The listing builds one solid part. Answer for the finished solid, in the listing's coordinates (mm). Face numbers are marked on the shaded views. Give positions to 0.01 mm unless a question says otherwise; leave off trailing zeros. Order: outer loops, then holes, each group sorted by start corner. A loop starts at its lowest first (then second) coordinate and runs counter-clockwise, first axis right, second up. Notation, with made-up numbers: (12, -26.75) - (39, -26.75) arc R29 ccw to (39, 12.25) - close; hole circle Ø4 at (-2.5, 80.5). An arc over 180 degrees is marked (long way). Answer as CSV lines item,"result". Start each with the question number.
1. Section A-A on y = 39 is taken. Give the vertices of the cut face in (x, z), and give its area (3 significant figures).
2. Flat-ended cylindrical pins translate along their axes: pin 1 (5.5 mm diameter, centred on x = -25.79, y = 74.34, fed in from +Z); pin 2 (7 mm diameter, centred on x = 26.21, y = -42.5, fed in from -Z). Find the tip coordinate at first contact, or state that the pin passes through.
3. Section B-B on z = 3 is taken. Give the vertices of the cut face in (x, y).
4. Section C-C on y = -69 is taken. Give the vertices of the cut face in (x, z), and give its area (3 significant figures).
5. Determine the mould class of the marked faces 1, 2 and 3 for opening direction X: +X half, -X half, draft (parallel to the pull), parting line (faces both ways), or undercut.
6. Consider line 1 along Y through (x, z) = (7, 7); line 2 along X through (y, z) = (32, 7.75); line 3 along Y through (x, z) = (-25.5, 7.5). Determine where each line is inside the solid, lowest interval first. Write a range as [from, to].
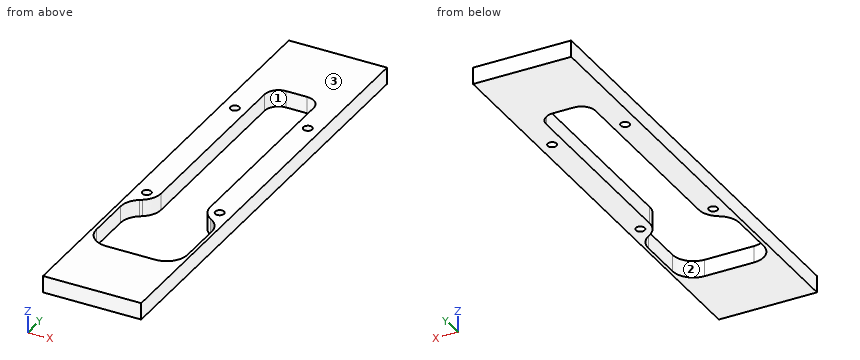
from build123d import *

# Parameters (mm, degrees)
F0_W     = 70
F0_H     = 326
F0_W_2   = 17
F0_H_2   = 17
F0_R     = 3.15
F1_DEPTH = 12
F2_R     = 15
F3_R     = 10


with BuildPart() as f1:
    # F0 (on Top) → F1 (new body)
    with BuildSketch(Plane.XY):
        Rectangle(F0_W, F0_H)
        Polygon((32.7086956522, -112.1642902674), (17.7086956522, -112.1642902674), (-17.2913043478, -112.1642902674), (-32.2913043478, -112.1642902674), (-32.2913043478, -57.1642902674), (-34.2913043478, -47.1642902674), (-34.2913043478, -32.1642902674), (-17.2913043478, -32.1642902674), (-17.2913043478, 65.8357097326), (-34.2913043478, 65.8357097326), (-34.2913043478, 82.8357097326), (-17.2913043478, 82.8357097326), (-17.2913043478, 107.8357097326), (17.7086956522, 107.8357097326), (17.7086956522, 82.8357097326), (34.7086956522, 82.8357097326), (34.7086956522, 65.8357097326), (17.7086956522, 65.8357097326), (17.7086956522, -32.1642902674), (34.7086956522, -32.1642902674), (34.7086956522, -47.1642902674), (32.7086956522, -57.1642902674), align=None, mode=Mode.SUBTRACT)
        Polygon((-34.2913043478, -47.1642902674), (-32.2913043478, -57.1642902674), (-17.2913043478, -47.1642902674), (-17.2913043478, -32.1642902674), (-34.2913043478, -32.1642902674), align=None)
        Polygon((-25.7913043478, -36.608650855), (-20.6913043478, -39.5531372279), (-20.6913043478, -45.4421099736), (-25.7913043478, -48.3865963465), (-30.8913043478, -45.4421099736), (-30.8913043478, -39.5531372279), align=None, mode=Mode.SUBTRACT)
        Polygon((17.7086956522, -47.1642902674), (32.7086956522, -57.1642902674), (34.7086956522, -47.1642902674), (34.7086956522, -32.1642902674), (17.7086956522, -32.1642902674), align=None)
        Polygon((31.3086956522, -45.4421099736), (26.2086956522, -48.3865963465), (21.1086956522, -45.4421099736), (21.1086956522, -39.5531372279), (26.2086956522, -36.608650855), (31.3086956522, -39.5531372279), align=None, mode=Mode.SUBTRACT)
        with Locations((-25.7913043478, 74.3357097326)):
            Rectangle(F0_W_2, F0_H_2)
        Polygon((-20.6913043478, 77.2801961054), (-20.6913043478, 71.3912233597), (-25.7913043478, 68.4467369868), (-30.8913043478, 71.3912233597), (-30.8913043478, 77.2801961054), (-25.7913043478, 80.2246824783), align=None, mode=Mode.SUBTRACT)
        with Locations((26.2086956522, 74.3357097326)):
            Rectangle(F0_W_2, F0_H_2)
        Polygon((31.3086956522, 71.3912233597), (26.2086956522, 68.4467369868), (21.1086956522, 71.3912233597), (21.1086956522, 77.2801961054), (26.2086956522, 80.2246824783), (31.3086956522, 77.2801961054), align=None, mode=Mode.SUBTRACT)
        Polygon((-20.6913043478, -45.4421099736), (-20.6913043478, -39.5531372279), (-25.7913043478, -36.608650855), (-30.8913043478, -39.5531372279), (-30.8913043478, -45.4421099736), (-25.7913043478, -48.3865963465), align=None)
        with Locations((-25.7913043478, -42.4976236008)):
            Circle(F0_R, mode=Mode.SUBTRACT)
        Polygon((21.1086956522, -45.4421099736), (26.2086956522, -48.3865963465), (31.3086956522, -45.4421099736), (31.3086956522, -39.5531372279), (26.2086956522, -36.608650855), (21.1086956522, -39.5531372279), align=None)
        with Locations((26.2086956522, -42.4976236008)):
            Circle(F0_R, mode=Mode.SUBTRACT)
        Polygon((-25.7913043478, 68.4467369868), (-20.6913043478, 71.3912233597), (-20.6913043478, 77.2801961054), (-25.7913043478, 80.2246824783), (-30.8913043478, 77.2801961054), (-30.8913043478, 71.3912233597), align=None)
        with Locations((-25.7913043478, 74.3357097326)):
            Circle(F0_R, mode=Mode.SUBTRACT)
        Polygon((21.1086956522, 71.3912233597), (26.2086956522, 68.4467369868), (31.3086956522, 71.3912233597), (31.3086956522, 77.2801961054), (26.2086956522, 80.2246824783), (21.1086956522, 77.2801961054), align=None)
        with Locations((26.2086956522, 74.3357097326)):
            Circle(F0_R, mode=Mode.SUBTRACT)
    extrude(amount=F1_DEPTH)

    # F2
    f2_edges = [f1.edges().sort_by_distance(p)[0] for p in [
        (-32.291304, -57.16429, 6),
        (-17.291304, -47.16429, 6),
        (17.708696, -47.16429, 6),
        (32.708696, -57.16429, 6),
        (32.708696, -112.16429, 6),
        (-32.291304, -112.16429, 6),
    ]]
    fillet(f2_edges, radius=F2_R)

    # F3
    f3_edges = [f1.edges().sort_by_distance(p)[0] for p in [
        (17.708696, 107.83571, 6),
        (-17.291304, 107.83571, 6),
    ]]
    fillet(f3_edges, radius=F3_R)


solid = f1.part
Checks:
1,outline,"(-35, 0) - (-17.29, 0) - (-17.29, 12) - (-35, 12) - close; (17.71, 0) - (35, 0) - (35, 12) - (17.71, 12) - close"
1,area,"420 mm²"
2,pin 1,"passes through"
2,pin 2,"stops at z = 0"
3,outline,"(-35, -163) - (35, -163) - (35, 163) - (-35, 163) - close; hole (-32.29, -97.16) arc R15 ccw to (-17.29, -112.16) - (17.71, -112.16) arc R15 ccw to (32.71, -97.16) - (32.71, -65.19) arc R15 ccw to (26.03, -52.71) - (24.39, -51.62) arc R15 cw to (17.71, -39.14) - (17.71, 97.84) arc R10 ccw to (7.71, 107.84) - (-7.29, 107.84) arc R10 ccw to (-17.29, 97.84) - (-17.29, -39.14) arc R15 cw to (-23.97, -51.62) - (-25.61, -52.71) arc R15 ccw to (-32.29, -65.19) - close; hole circle Ø6.3 at (-25.79, -42.5); hole circle Ø6.3 at (-25.79, 74.34); hole circle Ø6.3 at (26.21, -42.5); hole circle Ø6.3 at (26.21, 74.34)"
4,outline,"(-35, 0) - (-32.29, 0) - (-32.29, 12) - (-35, 12) - close; (32.71, 0) - (35, 0) - (35, 12) - (32.71, 12) - close"
4,area,"60.0 mm²"
5,face 1,"undercut"
5,face 2,"undercut"
5,face 3,"draft"
6,line 1,"y = [-163, -112.16], [107.84, 163]"
6,line 2,"x = [-35, -17.29], [17.71, 35]"
6,line 3,"y = [-163, -109.72], [-52.64, -45.63], [-39.36, 71.2], [77.47, 163]"
